Input: dimensioned drawing with shaded views. Units: mm. Origin: part minimum x, y, z. Round coordinates to 2 decimals unless told otherwise and drop trailing zeros. Order: outer loops, then holes, each group sorted by start corner. A loop starts at its lowest first (then second) coordinate and runs counter-clockwise, first axis right, second up. Notation, with made-up numbers: (39, 63) - (58, 63) arc R15 cw to (58, 84) - close; hole circle Ø2 at (46, -0.5). An arc over 180 degrees is marked (long way). Return JSON: item names as keys, results as strings. Group by question number.
1) Contact query for a flat-ended pin moving along its axis: P1, Ø5, axis at x = 59.8, z = 9, coming from the +Y side. Output: stop coordinate, or through.
2) Section C-C, the plane z = 6.5. Return loops of the section in (x, y), plus the area to 3 significant figures.
3) Section A-A, the plane x = 59.8. Return loops of the section in (y, z), plus the area to 3 significant figures.
4) Section B-B, the plane y = 3.25. Return loops of the section in (x, z), plus the area to 3 significant figures.
5) Ray query, line 1 (Z direction, x = 104.25, y = 6); line 2 (X direction, y = 6, z = 9.75); line 3 (X direction, y = 3.75, z = 7.75). Return the intervals inside material, ascending. Write a range as from..to.
6) Mould query, pull axis Z, two halves, no side actions, for the marked faces 1, 2 and 3. Classes: pulls with the +Z half, pulls with the -Z half, needs draft (parallel to the pull), parting line crosses it, or undercut.
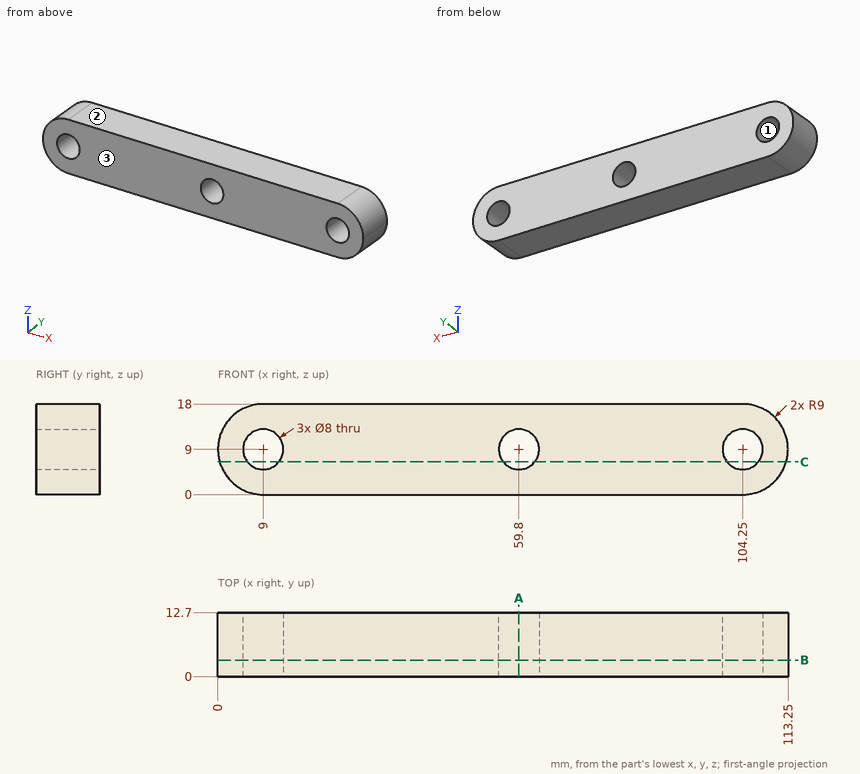
Geometry check:
{
 "1": {"P1": "through"},
 "2": {"outline": "(0.35, 0) - (5.88, 0) - (5.88, 12.7) - (0.35, 12.7) - close; (12.12, 0) - (56.68, 0) - (56.68, 12.7) - (12.12, 12.7) - close; (62.92, 0) - (101.13, 0) - (101.13, 12.7) - (62.92, 12.7) - close; (107.37, 0) - (112.9, 0) - (112.9, 12.7) - (107.37, 12.7) - close", "area": "1,190 mm2"},
 "3": {"outline": "(0, 0) - (12.7, 0) - (12.7, 5) - (0, 5) - close; (0, 13) - (12.7, 13) - (12.7, 18) - (0, 18) - close", "area": "127 mm2"},
 "4": {"outline": "(9, 0) - (104.25, 0) arc R9 ccw to (104.25, 18) - (9, 18) arc R9 ccw to start; hole circle Ø8 at (9, 9); hole circle Ø8 at (59.8, 9); hole circle Ø8 at (104.25, 9)", "area": "1,820 mm2"},
 "5": {"line 1": "0..5, 13..18", "line 2": "0.03..5.07, 12.93..55.87, 63.73..100.32, 108.18..113.22", "line 3": "0.09..5.2, 12.8..56, 63.6..100.45, 108.05..113.16"},
 "6": {"face 1": "undercut", "face 2": "pulls with the +Z half", "face 3": "needs draft"}
}
